```python
from build123d import *

# Parameters (mm, degrees)
F0_R     = 20
F1_DEPTH = 40
F3_DEPTH = 15


with BuildPart() as f1:
    # F0 (on Front) → F1 (new body)
    with BuildSketch(Plane.XZ):
        Circle(F0_R)
    extrude(amount=F1_DEPTH)

    # F2 (on Front) → F3 (cut)
    with BuildSketch(Plane.XZ):
        Polygon((3.95189, -14), (14.1003, -3.577563), (10.148411, 10.422437), (-3.95189, 14), (-14.1003, 3.577563), (-10.148411, -10.422437), align=None)
    extrude(amount=F3_DEPTH, mode=Mode.SUBTRACT)


solid = f1.part
```
Part model, mm, in its own coordinate system. A direction names the side the tool comes from. Coordinates: 2 decimals unless noted, no trailing zeros. Loops run counter-clockwise (first coordinate to the right, second up) from the corner with the lowest first, then second, coordinate; pieces in that order, holes last. Notation, with made-up numbers: (-9.75, -8.5) - (-4.75, -8.5) arc R10 cw to (-4.75, -3.5) - close; hole circle Ø5 at (23.25, 86.5). An arc over 180 degrees is marked (long way). Write item = value, one per line. Start each with the question number.
Item 1: Cut at B-B, the plane x = -5.5. Give the cut face in (y, z).
Item 2: Cut at A-A, the plane y = -8.5. Give the cut face in (x, z), and give its area (3 significant figures).
Item 3: 3-axis set-ups, long thin cutter, end or side, ignore diameter. For faces 1 (the flat face through (-8.955, -7.395, 8.862)), 2 (the flat face through (0, -40, 0)): which of +Z, -Z, +X, -X, +Y, -Y reach the whole face in a straight line?
Item 4: Wall check: L1, parallel to Y at x = 12, z = -3.5; L2, parallel to X at y = -19, z = 0.5; L3, parallel to X at y = -9, z = 1. Give the ranges that are in metal, low to high. Write a range as from..to.
Item 5: Flat gauge pins, fed straight in: pin 1 Ø5 at (x, y) = (2, -5) entering from +Z; pin 2 Ø12 at (y, z) = (-17, 1) entering from +X; pin 3 Ø6 at (y, z) = (-23.5, 9.5) entering from +X; pin 4 Ø3 at (y, z) = (-32.5, 7) entering from -X. Where does each tip first touch, or does it go through?
Item 6: Cut at C-C, the plane z = 4.5. Give the cut face in (x, y).
Item 7: Mould opens along X. For faces 3 (the flat face through (-12.152, -7.395, -3.324)), 4 (the flat face through (-9.2, 0, 9.2)), 5 (the cylindrical face through (-4.336, -19.72, -19.524)), 6 (the flat face through (0, -15, 0)) say: released by +X, released by -X, zero draft, split by the parting line, or undercut.
Item 8: Cut at D-D, the plane y = -18. Give the cut face in (x, z).
The answers:
q1.outline = (-40, -19.23) - (0, -19.23) - (0, -11.6) - (-15, -11.6) - (-15, 12.41) - (0, 12.41) - (0, 19.23) - (-40, 19.23) - close
q2.outline = circle Ø40 at (0, 0); hole (-14.1, 3.58) - (-10.15, -10.42) - (3.95, -14) - (14.1, -3.58) - (10.15, 10.42) - (-3.95, 14) - close
q2.area = 707 mm2
q3.face_1 = +Y
q3.face_2 = +Z, -Z, +X, -X, -Y
q4.L1 = -40..-15
q4.L2 = -19.99..19.99
q4.L3 = -19.97..-13.37, 12.81..19.97
q5.pin_1 = 20
q5.pin_2 = 20
q5.pin_3 = 18.91
q5.pin_4 = -19.23
q6.outline = (-19.49, -40) - (19.49, -40) - (19.49, 0) - (11.82, 0) - (11.82, -15) - (-13.2, -15) - (-13.2, 0) - (-19.49, 0) - close
q7.face_3 = undercut
q7.face_4 = zero draft
q7.face_5 = split by the parting line
q7.face_6 = undercut
q8.outline = circle Ø40 at (0, 0)
